```python
from build123d import *

# Parameters (mm, degrees)
SKETCH1_W           = 490
SKETCH1_H           = 1040
SKETCH1_W_2         = 430
SKETCH1_H_2         = 980
BOSS_EXTRUDE1_DEPTH = 370
SKETCH2_W           = 490
SKETCH2_H           = 1040
BOSS_EXTRUDE2_DEPTH = 30
SKETCH3_W           = 430
SKETCH3_H           = 160
BOSS_EXTRUDE3_DEPTH = 130
FILLET1_R           = 20
SKETCH5_W           = 30
SKETCH5_H           = 1010
CUT_EXTRUDE2_DEPTH  = 400
SKETCH7_R           = 3
BOSS_EXTRUDE4_DEPTH = 50
SKETCH8_W           = 84
SKETCH8_H           = 84
SKETCH8_W_2         = 80
SKETCH8_H_2         = 80
BOSS_EXTRUDE5_DEPTH = 300
SKETCH9_W           = 84
SKETCH9_H           = 82
CUT_EXTRUDE3_DEPTH  = 100


with BuildPart() as part:
    # Sketch1 → Boss-Extrude1 (new body)
    with BuildSketch(Plane.XY):
        Rectangle(SKETCH1_W, SKETCH1_H)
        Rectangle(SKETCH1_W_2, SKETCH1_H_2, mode=Mode.SUBTRACT)
    extrude(amount=BOSS_EXTRUDE1_DEPTH)

    # Sketch2 → Boss-Extrude2 (add)
    with BuildSketch(Plane(origin=(0, 0, 0), x_dir=(-1, 0, 0), z_dir=(0, 0, -1))):
        Rectangle(SKETCH2_W, SKETCH2_H)
    extrude(amount=BOSS_EXTRUDE2_DEPTH)

    # Sketch3 → Boss-Extrude3 (add)
    with BuildSketch(Plane.XY):
        with Locations((0, -410)):
            Rectangle(SKETCH3_W, SKETCH3_H)
    extrude(amount=BOSS_EXTRUDE3_DEPTH)

    # Fillet1
    fillet1_edges = [part.edges().sort_by_distance(p)[0] for p in [
        (0, -330, 130),
    ]]
    fillet(fillet1_edges, radius=FILLET1_R)

    # Sketch5 → Cut-Extrude2 (cut)
    with BuildSketch(Plane.XY.offset(370)):
        with Locations((-230, 15)):
            Rectangle(SKETCH5_W, SKETCH5_H)
    extrude(amount=-CUT_EXTRUDE2_DEPTH, mode=Mode.SUBTRACT)

    # Sketch7 → Boss-Extrude4 (add)
    with BuildSketch(Plane.ZY.offset(-215)):
        with Locations((160, 280)):
            Circle(SKETCH7_R)
        with Locations((160, 160)):
            Circle(SKETCH7_R)
        with Locations((160, 40)):
            Circle(SKETCH7_R)
        with Locations((160, -80)):
            Circle(SKETCH7_R)
        with Locations((160, -200)):
            Circle(SKETCH7_R)
    extrude(amount=BOSS_EXTRUDE4_DEPTH)

    # Sketch8 → Boss-Extrude5 (add)
    with BuildSketch(Plane.XY):
        with Locations((-15, 450)):
            Rectangle(SKETCH8_W, SKETCH8_H)
        with Locations((-15, 450)):
            Rectangle(SKETCH8_W_2, SKETCH8_H_2, mode=Mode.SUBTRACT)
    extrude(amount=BOSS_EXTRUDE5_DEPTH)

    # Sketch9 → Cut-Extrude3 (cut)
    with BuildSketch(Plane.XY):
        with Locations((-15, 449)):
            Rectangle(SKETCH9_W, SKETCH9_H)
    extrude(amount=CUT_EXTRUDE3_DEPTH, mode=Mode.SUBTRACT)


solid = part.part
```
Model file for the job. Use its own axes, mm. A direction names the side the tool comes from. Give positions to 0.01 mm unless a question says otherwise; leave off trailing zeros. Write each loop counter-clockwise with the first axis right and the second up, starting at its lowest first coordinate (ties: lowest second). Pieces come first, ordered by that corner, then holes. Notation, with made-up numbers: M 83,38.25 L 102,38.25 A21 ccw 102,44.25 Z; hole C 12.5,-3 d2. An arc over 180 degrees is marked long. Use a Markdown table: item, result.
1) Pull direction Z, two halves, no side cores. Call faces 1 (the flat face through (217, 2, 370)), 2 (the flat face through (-57, 448, 199)), 3 (the flat face through (-15.2, 409.7, 100)): +Z half, -Z half, draft (parallel to the pull), parting line (faces both ways), or undercut.
Responses:
| item | result |
|---|---|
| face 1 | +Z half |
| face 2 | draft |
| face 3 | undercut |
2) Cut at D-D (z = 33.5). List the corners of the cut face in (x, y), and give its area (3 significant figures).
Responses:
| item | result |
|---|---|
| outline | M -245,-520 L 245,-520 L 245,520 L -215,520 L -215,490 L 215,490 L 215,-330 L -215,-330 L -215,-490 L -245,-490 Z |
| area | 127,000 mm2 |
3) Drill centre lines: line 1 (X direction, y = 464, z = 280); line 2 (Y direction, x = -3.5, z = 132.5); line 3 (Y direction, x = 143, z = 52). Where is each one in solid material? Low to high. Write a range as from..to.
Responses:
| item | result |
|---|---|
| line 1 | x = -57..-55, 25..27, 215..245 |
| line 2 | y = -520..-490, 408..410, 490..520 |
| line 3 | y = -520..-330, 490..520 |
4) Cut at B-B (z = 249). List the corners of the cut face in (x, y).
Responses:
| item | result |
|---|---|
| outline | M -245,-520 L 245,-520 L 245,520 L -215,520 L -215,490 L -57,490 L -57,408 L 27,408 L 27,490 L 215,490 L 215,-490 L -245,-490 Z; hole M -55,410 L 25,410 L 25,490 L -55,490 Z |
5) Tool access for faces 4 (the flat face through (-16, 408, 199)), 5 (the flat face through (-215, -25, -7)), 6 (the flat face through (25, 449, 199)): list every direction of +Z, -Z, +X, -X, +Y, -Y with a clear straight run to the whole face (end or side of a thin tool).
Responses:
| item | result |
|---|---|
| face 4 | +Z, -X |
| face 5 | +Z, -Z, -X, +Y |
| face 6 | +Z |
6) Cut at C-C (y = -363). List the corners of the cut face in (x, z), and give its area (3 significant figures).
Responses:
| item | result |
|---|---|
| outline | M -215,-30 L 245,-30 L 245,370 L 215,370 L 215,130 L -215,130 Z |
| area | 80,800 mm2 |
7) Cut at A-A (x = 5). List the corners of the cut face in (y, z).
Responses:
| item | result |
|---|---|
| outline | M -520,-30 L 520,-30 L 520,370 L 490,370 L 490,0 L -330,0 L -330,110 A20 ccw -350,130 L -490,130 L -490,370 L -520,370 Z; M 408,100 L 410,100 L 410,300 L 408,300 Z |
8) Pin check, flat tips, straight feed: pin 1 (6.5 mm diameter, centred on y = 161, z = 160, fed in from -X); pin 2 (12 mm diameter, centred on x = 155, y = -141, fed in from +Z); pin 3 (4 mm diameter, centred on y = -268.5, z = 23, fed in from -X). Stop position of each tip, or through.
Responses:
| item | result |
|---|---|
| pin 1 | stops at x = 165 |
| pin 2 | stops at z = 0 |
| pin 3 | stops at x = 215 |
